Read the model definition and answer for the solid it produces. Units are mm, in the model's axes. Face numbers are marked on the shaded views. A direction names the side the tool comes from. Coordinates: 2 decimals unless noted, no trailing zeros. Order: outer loops, then holes, each group sorted by start corner. A loop starts at its lowest first (then second) coordinate and runs counter-clockwise, first axis right, second up. Notation, with made-up numbers: (77, 23) -> (84, 23) arc R27 ccw to (84, 57) -> close; hole circle Ø6 at (33, 60). An arc over 180 degrees is marked (long way). Return JSON: item names as keys, results as strings. Group by question number.
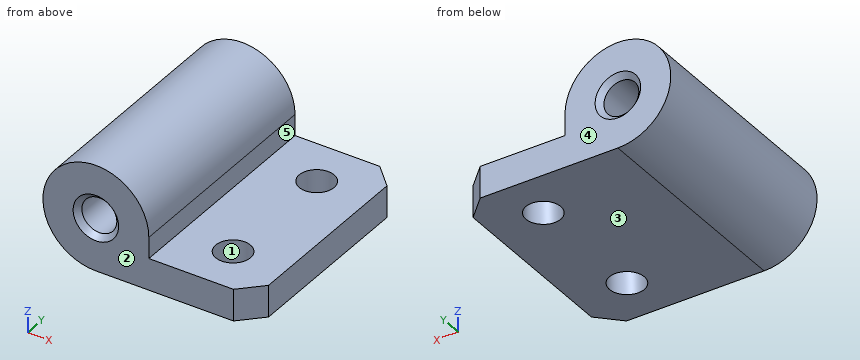
```python
from build123d import *

# Parameters (mm, degrees)
SKETCH_R        = 1.65
PAD_DEPTH       = 10.5
CHAMFER_SIZE    = 0.5
CHAMFER001_SIZE = 2
SKETCH001_R     = 1.65
POCKET_DEPTH    = 3.001


with BuildPart() as part:
    # Sketch → Pad (new body, symmetric)
    with BuildSketch(Plane.XZ):
        with BuildLine():
            ThreePointArc((5, 4.999972), (-3.535524, 8.535544), (0, 0))
            Line((0, 0), (15, 0))
            Line((15, 0), (15, 3))
            Line((15, 3), (5, 3))
            Line((5, 3), (5, 4.999972))
        make_face()
        with Locations((0, 5)):
            Circle(SKETCH_R, mode=Mode.SUBTRACT)
    extrude(amount=PAD_DEPTH, both=True)

    # Chamfer
    chamfer_edges = [part.edges().sort_by_distance(p)[0] for p in [
        (-1.65, -10.5, 5),
        (-1.65, 10.5, 5),
    ]]
    chamfer(chamfer_edges, length=CHAMFER_SIZE)

    # Chamfer001
    chamfer001_edges = [part.edges().sort_by_distance(p)[0] for p in [
        (15, 10.5, 1.5),
        (15, -10.5, 1.5),
    ]]
    chamfer(chamfer001_edges, length=CHAMFER001_SIZE)

    # Sketch001 → Pocket (cut, through all)
    with BuildSketch(Plane(origin=(0, 0, 3), x_dir=(-1, 0, 0), z_dir=(0, 0, 1))):
        with Locations((-10, 6)):
            Circle(SKETCH001_R)
        with Locations((-10, -6)):
            Circle(SKETCH001_R)
    extrude(amount=-POCKET_DEPTH, mode=Mode.SUBTRACT)


solid = part.part
```
1. Straight lines are drawn through the part: L1, parallel to Y at x = 10, z = 0.75; L2, parallel to Z at x = 7.25, y = 4.75; L3, parallel to Z at x = 0, y = 2.5. For each, find the intervals that lie inside material, in ascending order.
2. Find section C-C on z = 1. Determine the outline of the cut face in (x, y).
3. Which of the six approach directions +Z, -Z, +X, -X, +Y, -Y give full straight-line access (tool end or side, diameter ignored) to the marked faces 4 and 5?
4. Given pin 1 (1.5 mm diameter, centred on x = 9.5, y = 8, fed in from +Z); pin 2 (3 mm diameter, centred on x = 2.5, y = 3.5, fed in from +Z); pin 3 (1 mm diameter, centred on y = -3.5, z = 7, fed in from -X), each flat-ended and moving along its own axis, determine where each tip first touches the part or whether it passes through.
5. Find section A-A on y = 6. Determine the outline of the cut face in (x, z), and give its area (3 significant figures).
6. Find section B-B on x = 10. Determine the outline of the cut face in (y, z), and give its area (3 significant figures).
7. Find section D-D on y = -2.5. Determine the outline of the cut face in (x, z), and give its area (3 significant figures).
8. For a pull along Y with two mould halves and no side action, classify the marked faces 1, 2 and 3 as released by +Y, released by -Y, zero draft, split by the parting line, or undercut.
Result:
{
 "1": {"L1": "-10.5 to -7.65, -4.35 to 4.35, 7.65 to 10.5", "L2": "0 to 3", "L3": "0 to 3.35, 6.65 to 10"},
 "2": {"outline": "(-3, -10.5) -> (13, -10.5) -> (15, -8.5) -> (15, 8.5) -> (13, 10.5) -> (-3, 10.5) -> close; hole circle Ø3.3 at (10, -6); hole circle Ø3.3 at (10, 6)"},
 "3": {"face 4": "+Z, -Z, +X, -X, +Y", "face 5": "+Z, +X, +Y, -Y"},
 "4": {"pin 1": "z = 3", "pin 2": "z = 9.9", "pin 3": "x = -4.77"},
 "5": {"outline": "(0, 0) -> (8.35, 0) -> (8.35, 3) -> (5, 3) -> (5, 5) arc R5 ccw (long way) to start; (11.65, 0) -> (15, 0) -> (15, 3) -> (11.65, 3) -> close; hole circle Ø3.3 at (0, 5)", "area": "95.5 mm^2"},
 "6": {"outline": "(-10.5, 0) -> (-7.65, 0) -> (-7.65, 3) -> (-10.5, 3) -> close; (-4.35, 0) -> (4.35, 0) -> (4.35, 3) -> (-4.35, 3) -> close; (7.65, 0) -> (10.5, 0) -> (10.5, 3) -> (7.65, 3) -> close", "area": "43.2 mm^2"},
 "7": {"outline": "(0, 0) -> (15, 0) -> (15, 3) -> (5, 3) -> (5, 5) arc R5 ccw (long way) to start; hole circle Ø3.3 at (0, 5)", "area": "105 mm^2"},
 "8": {"face 1": "undercut", "face 2": "released by -Y", "face 3": "zero draft"}
}
